Autodesk Inventor part; units mm, degrees
ref_plane "Plano de trabajo1" through (0, 95.1, 0) normal (0, -1, 0) x (1, 0, 0)
ref_plane "Plano de trabajo2" through (0, 106.9, 0) normal (0, 1, 0) x (1, 0, 0)
ref_plane "YZ Plane" through (0, 0, 0) normal (1, 0, 0) x (0, 1, 0)
sketch "Boceto1" plane through (0, 0, 0) normal (0, 1, 0) x (-1, 0, 0)
  circle A0 centre (0, 0) radius 7.275
  circle A1 centre (0, 0) radius 8.7
  dimension "d0" = 14.55
  dimension "d1" = 17.4
extrude "Extrusión1" add sketch "Boceto1" along normal blind 5.9 contours A0
sketch "Boceto2" plane through (0, 5.9, 0) normal (0, 1, 0) x (1, 0, 0)
  circle A0 centre (0, 0) radius 8.7
  dimension "d5" = 17.4
ref_plane "Plano de trabajo1" through (0, 95.1, 0) normal (0, -1, 0) x (1, 0, 0)
sketch "Boceto3" plane through (0, 95.1, 0) normal (0, -1, 0) x (1, 0, 0)
  circle A0 centre (0, 0) radius 8.115
  dimension "d7" = 16.23
loft "Solevación1" add profiles "Boceto3", "Boceto2"
sketch "Boceto4" plane through (0, 0, 0) normal (0, -1, 0) x (1, 0, 0)
  circle A0 centre (0, 0) radius 7.275
  circle A1 centre (0, 0) radius 6.515
  dimension "d12" = 13.03
extrude "Extrusión2" cut sketch "Boceto4" against normal blind 1.08 contours A1
sketch "Boceto5" plane through (0, 95.1, 0) normal (0, 1, 0) x (1, 0, 0)
  circle A0 centre (0, 0) radius 7.21
  dimension "d15" = 14.42
extrude "Extrusión3" add sketch "Boceto5" along normal blind 2.65
ref_plane "Plano de trabajo2" through (0, 106.9, 0) normal (0, 1, 0) x (1, 0, 0)
sketch "Boceto6" plane through (0, 106.9, 0) normal (0, 1, 0) x (1, 0, 0)
  circle A0 centre (0, 0) radius 3.95
  dimension "d19" = 7.9
loft "Solevación2" add profiles "Boceto6" section 2 edges at (-7.21, 97.75, 0)
sketch "Boceto7" plane through (0, 106.9, 0) normal (0, 1, 0) x (1, 0, 0)
  circle A0 centre (0, 0) radius 3.95
extrude "Extrusión4" add sketch "Boceto7" along normal blind 6.58
sketch "Boceto8" plane through (0, 113.48, 0) normal (0, 1, 0) x (1, 0, 0)
  line L0 (1.8, 2.78) -> (-1.8, 2.78)
  line L1 (-1.8, 2.78) -> (-1.8, -2.78)
  line L2 (-1.8, -2.78) -> (1.8, -2.78)
  line L3 (1.8, -2.78) -> (1.8, 2.78)
  circle A0 centre (0, 0) radius 3.95
  line L4 (1.8, 2.78) -> (-1.8, -2.78) construction
  line L5 (-1.8, 2.78) -> (1.8, -2.78) construction
  dimension "d26" = 3.6
  dimension "d27" = 5.56
extrude "Extrusión5" add sketch "Boceto8" along normal blind 8.65 contours L3 L2 L1 L0
sketch "Boceto9" plane through (-1.8, 113.48, -2.78) normal (-1, 0, 0) x (0, 0, 1)
  line L0 (0, 0) -> (0, 8.65)
  line L1 (0, 0) -> (0, 7)
  line L2 (0, 8.65) -> (5.56, 8.65)
  line L3 (0, 7) -> (5.56, 8.65)
  point P0 (2.78, -113.48)
  dimension "d30" = 7
extrude "Extrusión6" cut sketch "Boceto9" against normal blind 8.65
properties part number "MARCADOR"
Can you work these out from the model? Positions are in its coordinate system, mm. A direction names the side the tool comes from. Coordinates: 2 decimals unless noted, no trailing zeros. Write each loop counter-clockwise with the first axis right and the second up, starting at its lowest first coordinate (ties: lowest second). Pieces come first, ordered by that corner, then holes. Notation, with made-up numbers: (-15.75, -0.75) -> (-1.75, -0.75) arc R24 cw to (-1.75, 31.25) -> close; hole circle Ø2 at (-6.5, 1.5). An arc over 180 degrees is marked (long way). Write each question's results on one line, items separated by ' | '. Start each with the question number.
Q1. We'd pull the mould along X, two halves only. Please class faces 5 (the face through (7, 0, 1)), 6 (the face through (-1.8, 118, 0)), 7 (the face through (0, 1.08, 0)), 8 (the face through (-1.41, 0.53, -6.36)): +X half, -X half, draft (parallel to the pull), parting line (faces both ways), or undercut.
Q2. Imagine slicing it at A-A (y = 109.5). Write out the boundary of the cut face in (x, z), then the cut area to 3 significant figures.
Q3. On a 3-axis mill with a long thin cutter (end or side, diameter ignored), from which of +Z, -Z, +X, -X, +Y, -Y can I reach the whole of each face in a straight line? I mean faces 1 (the face through (1.8, 118, 0)), 2 (the face through (-6, 96, -4)), 3 (the face through (0.947, 2.909, -7.213)), 4 (the face through (0, 117, -2.78)). Say none if no direction works.
Q4. Imagine slicing it at B-B (y = 64.5). Write out the boundary of the cut face in (x, z).
Q5. If I drill on probe 1 along Z at (x, y) = (0, 0.75) (3 decimals); probe 2 along X at (y, z) = (46.5, 2.25); probe 3 along Y at (x, z) = (-4.75, 5.75), over which ranges is the centre line in solid material (lowest first)?
Q6. I'm going to push flat-ended pins straight in: pin 1 (1.1 mm diameter, centred on x = 0.5, y = 115.5, fed in from -Z); pin 2 (8 mm diameter, centred on x = 4, z = 1.5, fed in from +Y); pin 3 (1.7 mm diameter, centred on y = 118.5, z = -1, fed in from -X); pin 4 (4.5 mm diameter, centred on y = 116, z = 0.5, fed in from +X). Where does each tip first touch, or does it pass through?
Taken from the geometry:
1) face 5: draft | face 6: -X half | face 7: undercut | face 8: undercut
2) outline: circle Ø7.9 at (0, 0) | area: 49.0 mm^2
3) face 1: +Z, -Z, +X, +Y | face 2: +Y | face 3: -Y | face 4: -Z, +X, -X, +Y
4) outline: circle Ø16.63 at (0, 0)
5) probe 1: z = -7.275 to -6.515, 6.515 to 7.275 | probe 2: x = -8.13 to 8.13 | probe 3: y = 5.9 to 95.1
6) pin 1: stops at z = -2.78 | pin 2: stops at y = 122.13 | pin 3: stops at x = -1.8 | pin 4: stops at x = 1.8
